Autodesk Inventor part; units mm, degrees
ref_plane "YZ Plane" through (0, 0, 0) normal (1, 0, 0) x (0, 1, 0)
ref_plane "XZ Plane" through (0, 0, 0) normal (0, 1, 0) x (-1, 0, 0)
ref_plane "XY Plane" through (0, 0, 0) normal (0, 0, 1) x (1, 0, 0)
sketch "Sketch1" plane through (0, 0, 0) normal (0, 1, 0) x (-1, 0, 0)
  circle A0 centre (0, 0) radius 15
  dimension "d0" = 30
extrude "Extrusion1" add sketch "Sketch1" along normal blind 2050
sketch "Sketch2" plane through (0, 0, 0) normal (0, -1, 0) x (1, 0, 0)
  circle A0 centre (0, 0) radius 15
  line L0 (0, 15) -> (0, -15)
extrude "Extrusion2" add sketch "Sketch2" along normal blind 0.1 contours A0 L0 picked at (3.1174, 3.9092)
sketch "Sketch4" plane through (0, 0, 0) normal (1, 0, 0) x (0, 1, 0)
  line L0 (2050, -15) -> (2050, 15)
  line L1 (0, 15) -> (0, -15)
  line L2 (0, 15) -> (-0.1, 15)
  line L3 (-0.1, -15) -> (-0.1, 15)
  line L4 (0, -15) -> (-0.1, -15)
  line L5 (-0.1, 15) -> (2050, 15)
  line L6 (-0.1, -15) -> (2050, -15)
  circle A0 centre (400, 0) radius 5
  circle A1 centre (800, 0) radius 5
  circle A2 centre (1250, 0) radius 5
  circle A3 centre (1650, 0) radius 5
  line L7 (1025, 15) -> (1025, -15)
  point P0 (0, 0)
  dimension "d9" = 1025
  dimension "d10" = 400
  dimension "d11" = 400
  dimension "d12" = 400
  dimension "d13" = 400
  dimension "d14" = 10
  dimension "d15" = 10
  dimension "d16" = 10
  dimension "d17" = 10
extrude "Extrusion3" add sketch "Sketch4" against normal blind 40 contours A0 | A1 | A2 | A3
properties part number "X_Rail-Rod-Rev1"
Verification items for the finished model (mm, model axes). Give positions to 0.01 mm unless a question says otherwise; leave off trailing zeros. Order: outer loops, then holes, each group sorted by start corner. A loop starts at its lowest first (then second) coordinate and runs counter-clockwise, first axis right, second up. Notation, with made-up numbers: M 80,62 L 105,62 A34 cw 105,93 Z; hole C 5,14.5 d8. An arc over 180 degrees is marked long. Answer as a JSON object with one key per item and string values. Group by question number.
1) Cross-section at A-A (z = 0). Enter the section's corners in (x, y).
2) Cross-section at B-B (y = 1772). Enter the section's corners in (x, z).
3) Depth check by flat-ended pin: pin 1 Ø6 at (x, y) = (4.5, 603) entering from +Z; pin 2 Ø5 at (x, y) = (-18, 997) entering from +Z; pin 3 Ø6 at (x, y) = (-32.5, 1655.5) entering from +Z; pin 4 Ø8 at (x, y) = (2, 247.5) entering from +Z. Enter the tip coordinate at first touch or a pass-through.
4) Scan lines: line 1 along Y through (x, z) = (-31.5, 1.5); line 2 along Y through (x, z) = (-33, 2); line 3 along X through (y, z) = (1887, -0.5). Record each from-to range of solid material in increasing order. Write a range as [from, to].
Result sheet:
{
 "1": {"outline": "M -40,395 L -15,395 L -15,0 L 0,0 L 0,-0.1 L 15,-0.1 L 15,2050 L -15,2050 L -15,1655 L -40,1655 L -40,1645 L -15,1645 L -15,1255 L -40,1255 L -40,1245 L -15,1245 L -15,805 L -40,805 L -40,795 L -15,795 L -15,405 L -40,405 Z"},
 "2": {"outline": "C 0,0 d30"},
 "3": {"pin 1": "stops at z = 14.92", "pin 2": "passes through", "pin 3": "stops at z = 4.33", "pin 4": "stops at z = 15"},
 "4": {"line 1": "y = [395.23, 404.77], [795.23, 804.77], [1245.23, 1254.77], [1645.23, 1654.77]", "line 2": "y = [395.42, 404.58], [795.42, 804.58], [1245.42, 1254.58], [1645.42, 1654.58]", "line 3": "x = [-14.99, 14.99]"}
}
